Could you check a few things on this model? Use its own coordinates, in mm. A direction names the side the tool comes from. Give positions to 0.01 mm unless a question says otherwise; leave off trailing zeros. Loops run counter-clockwise (first coordinate to the right, second up) from the corner with the lowest first, then second, coordinate; pieces in that order, holes last. Notation, with made-up numbers: M -8,66.5 L -3,66.5 A7 ccw -3,76.5 Z; hole C -8,18.5 d11. An arc over 180 degrees is marked long. Answer in a Markdown table with one row per item. Add a question column.
```python
from build123d import *

# Parameters (mm, degrees)
SKETCH_1_R      = 2.1
EXTRUDE_1_DEPTH = 3
FILLET_1_R      = 5


with BuildPart() as part:
    # 草图1 → 凸台-拉伸1 (new body)
    with BuildSketch(Plane(origin=(0, 0, 0), x_dir=(0, 0, -1), z_dir=(1, 0, 0))):
        Polygon((-10, 10), (-10, 50), (10, 50), (10, 10), (30, 10), (30, -10), (-30, -10), (-30, 10), align=None)
        with Locations((-20, 0)):
            Circle(SKETCH_1_R, mode=Mode.SUBTRACT)
        Circle(SKETCH_1_R, mode=Mode.SUBTRACT)
        with Locations((20, 0)):
            Circle(SKETCH_1_R, mode=Mode.SUBTRACT)
        with Locations((0, 20)):
            Circle(SKETCH_1_R, mode=Mode.SUBTRACT)
        with Locations((0, 40)):
            Circle(SKETCH_1_R, mode=Mode.SUBTRACT)
    extrude(amount=EXTRUDE_1_DEPTH)

    # 圆角1
    fillet_1_edges = [part.edges().sort_by_distance(p)[0] for p in [
        (1.5, -10, -30),
        (1.5, -10, 30),
        (1.5, 10, 30),
        (1.5, 10, 10),
        (1.5, 50, 10),
        (1.5, 50, -10),
        (1.5, 10, -10),
        (1.5, 10, -30),
    ]]
    fillet(fillet_1_edges, radius=FILLET_1_R)


solid = part.part
```
Item 1: Suppose I cut it at C-C (x = 1.6). List the corners of the cut face in (y, z) for me, then the cut area to 3 significant figures.
Item 2: I need wall thicknesses on L1, parallel to Y at x = 1.3, z = 0; L2, parallel to Y at x = 1.9, z = -20; L3, parallel to Y at x = 2.65, z = -24. Which ranges of each line are inside material? Lowest first, please.
Item 3: For P1, Ø0.9, axis at x = 1, y = 35, coming from the -Z side; P2, Ø1.5, axis at x = 2.5, z = 22, coming from the +Y side; P3, Ø0.9, axis at x = 1.5, y = 33, coming from the +Z side, each with a flat end and sliding along its axis, tell me the tip position at first contact or that it passes through.
Item 4: Suppose I cut it at A-A (y = 40). List the corners of the cut face in (x, z) for me.
Item 5: Suppose I cut it at D-D (y = 0). List the corners of the cut face in (x, z) for me.
Item 6: If we mould it in two halves opening along Y, with no side actions, what happens to faces 3 (the face through (0, 14, 0)), 4 (the face through (1.48, 37.95, 0.46)), 5 (the face through (2, -9, -28)), 6 (the face through (2, 12, -11))? For each: +Y half, -Y half, draft (parallel to the pull), parting line (faces both ways), or undercut.
Item 7: For faces 1 (the face through (2, -8, 29)), 2 (the face through (1, 10, -20)), which set-ups out of +Z, -Z, +X, -X, +Y, -Y let a thin tool reach every point of the face, with its end or its side?
Values found:
| question | item | result |
|---|---|---|
| 1 | outline | M -10,-25 A5 ccw -5,-30 L 5,-30 A5 ccw 10,-25 L 10,-15 A5 cw 15,-10 L 45,-10 A5 ccw 50,-5 L 50,5 A5 ccw 45,10 L 15,10 A5 cw 10,15 L 10,25 A5 ccw 5,30 L -5,30 A5 ccw -10,25 Z; hole C 0,-20 d4.2; hole C 0,0 d4.2; hole C 0,20 d4.2; hole C 20,0 d4.2; hole C 40,0 d4.2 |
| 1 | area | 1,910 mm² |
| 2 | L1 | -10 to -2.1, 2.1 to 17.9, 22.1 to 37.9, 42.1 to 50 |
| 2 | L2 | -10 to -2.1, 2.1 to 10 |
| 2 | L3 | -10 to 10 |
| 3 | P1 | z = -10 |
| 3 | P2 | y = 10 |
| 3 | P3 | z = 10 |
| 4 | outline | M 0,-10 L 3,-10 L 3,-2.1 L 0,-2.1 Z; M 0,2.1 L 3,2.1 L 3,10 L 0,10 Z |
| 5 | outline | M 0,-30 L 3,-30 L 3,-22.1 L 0,-22.1 Z; M 0,-17.9 L 3,-17.9 L 3,-2.1 L 0,-2.1 Z; M 0,2.1 L 3,2.1 L 3,17.9 L 0,17.9 Z; M 0,22.1 L 3,22.1 L 3,30 L 0,30 Z |
| 6 | face 3 | draft |
| 6 | face 4 | undercut |
| 6 | face 5 | -Y half |
| 6 | face 6 | +Y half |
| 7 | face 1 | +Z, +X, -X, -Y |
| 7 | face 2 | -Z, +X, -X, +Y |
